Can you work these out from the model? Positions are in its coordinate system, mm. Coordinates: 2 decimals unless noted, no trailing zeros. Order: outer loops, then holes, each group sorted by start corner. A loop starts at its lowest first (then second) coordinate and runs counter-clockwise, first axis right, second up. Notation, with made-up numbers: (15, -13.5) -> (74, -13.5) arc R18 ccw to (74, 16.5) -> close; hole circle Ø11 at (-25, 10.5). An arc over 180 degrees is marked (long way). Answer as CSV lines item,"result".
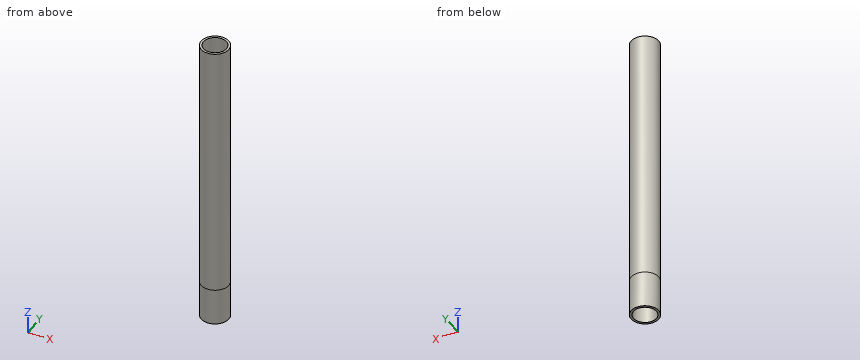
from build123d import *

# Parameters (mm, degrees)
F0_R     = 9.525
F0_R_2   = 7.9375
F1_DEPTH = 152.4
F2_DEPTH = 25.4
F3_DEPTH = 25.4


with BuildPart() as f1:
    # F0 (on Top) → F1 (new body)
    with BuildSketch(Plane.XY):
        Circle(F0_R)
        Circle(F0_R_2, mode=Mode.SUBTRACT)
    extrude(amount=F1_DEPTH)

    # F2 (add): a face of the model
    f2_faces = [f1.faces().sort_by_distance(p)[0] for p in [
        (-9.2555923164, 0, 152.4),
    ]]
    extrude(f2_faces, amount=F2_DEPTH)

    # F3 (add): a face of the model
    f3_faces = [f1.faces().sort_by_distance(p)[0] for p in [
        (-9.2555923164, 0, 0),
    ]]
    extrude(f3_faces, amount=F3_DEPTH)


solid = f1.part
Q1. For P1, Ø5, axis at x = 0.5, z = 16, coming from the +Y side (3 decimals); P2, Ø9.5, axis at x = 0, y = 0, coming from the +Z side; P3, Ø6, axis at x = 4.5, z = 99.5, coming from the -Y side; P4, Ø8, axis at x = -6, z = 0, coming from the +Y side, each with a flat end and sliding along its axis, tell me the tip position at first contact or that it passes through.
Solution:
P1,"y = 9.525"
P2,"through"
P3,"y = -9.41"
P4,"y = 9.31"
Q2. Imagine slicing it at A-A (y = 0). List the corners of the cut face in (x, z) for me (1 decimal), and give its area (3 significant figures).
Solution:
outline,"(-9.5, -25.4) -> (-7.9, -25.4) -> (-7.9, 177.8) -> (-9.5, 177.8) -> close; (7.9, -25.4) -> (9.5, -25.4) -> (9.5, 177.8) -> (7.9, 177.8) -> close"
area,"645 mm2"
Q3. If I drill on line 1 (Y direction, x = 0, z = -12.5) (1 decimal); line 2 (X direction, y = -0.5, z = 18); line 3 (X direction, y = 5.25, z = 28.5), over which ranges is the centre line in solid material (lowest first)?
Solution:
line 1,"-9.5 to -7.9, 7.9 to 9.5"
line 2,"-9.51 to -7.92, 7.92 to 9.51"
line 3,"-7.95 to -5.95, 5.95 to 7.95"
